Check sheet for the modelled part. Datum: model origin and axes. Units: mm. A direction names the side the tool comes from. Give positions to 0.01 mm unless a question says otherwise; leave off trailing zeros. Loops run counter-clockwise (first coordinate to the right, second up) from the corner with the lowest first, then second, coordinate; pieces in that order, holes last. Notation, with made-up numbers: M -28.5,18 L 23.5,18 A27 cw 23.5,54 Z; hole C -20,68.5 d3. An arc over 180 degrees is marked long. Write each question's results on one line, items separated by ' | '. Start each with the question number.
1. Go/stop test with flat-tipped pins: pin 1 (2.5 mm diameter, centred on x = -27, y = 6.5, fed in from -Z); pin 2 (0.6 mm diameter, centred on y = 6, z = -4, fed in from -X); pin 3 (6.5 mm diameter, centred on x = 27.5, y = 6, fed in from -Z). Record where each tip stops, or that it passes through.
2. Material ranges on line 1 along Y through (x, z) = (27.5, 5); line 2 along Z through (x, y) = (0, 8.75); line 3 along X through (y, z) = (4.75, -0.5), recorded low to high.
3. Sectioned sample at A-A on y = 7.5. Give the number of separate pieces and of enclosed holes in the cut face, and give its area (3 significant figures).
4. Tool access check on faces 5 (the cylindrical face through (-19.287, 0.752, -3.754)), 6 (the cylindrical face through (19.287, 0.752, -3.746)), 7 (the cylindrical face through (0, 14, -6)), 8 (the flat face through (0, 7, 1.5)), 9 (the flat face through (25.8, 5.8, 3.4)). Record the directions out of +Z, -Z, +X, -X, +Y, -Y that give a thin tool (end or side, any length) a straight path to the whole face; none if there is none.
5. Draft check along X on faces 1 (the flat face through (31, 5, -1)), 2 (the flat face through (35, 7, 3)), 3 (the cylindrical face through (-19, 8, -6)), 4 (the flat face through (-10, 7, 0)). Enter one of: pulls with the +X half, pulls with the -X half, needs draft (parallel to the pull), parting line crosses it, or undercut.
6. Sectioned sample at C-C on z = 5. Record the cut outline in (x, y), and give its area (3 significant figures).
7. Sectioned sample at D-D on y = 1.25. Record the cut outline in (x, z).
8. Sectioned sample at B-B on x = 27.5. Record the cut outline in (y, z).
```python
from build123d import *

# Parameters (mm, degrees)
SKETCH1_W                                           = 20
SKETCH1_H                                           = 3
BOSS_EXTRUDE1_DEPTH                                 = 15
CBORE_FOR_M4_HEX_SOCKET_HEAD_CAP_SCREW1_D           = 4.5
CBORE_FOR_M4_HEX_SOCKET_HEAD_CAP_SCREW1_CBORE_D     = 8
CBORE_FOR_M4_HEX_SOCKET_HEAD_CAP_SCREW1_CBORE_DEPTH = 4.4
FILLET1_R                                           = 2.5


with BuildPart() as part:
    # Sketch1 → Boss-Extrude1 (new body)
    with BuildSketch(Plane(origin=(0, 0, 0), x_dir=(1, 0, 0), z_dir=(0, 1, 0))):
        Polygon((-20, 6.5), (20, 6.5), (20, 1), (35, 1), (35, -8), (-35, -8), (-35, 1), (-20, 1), align=None)
        Rectangle(SKETCH1_W, SKETCH1_H, mode=Mode.SUBTRACT)
    extrude(amount=BOSS_EXTRUDE1_DEPTH)

    # CBORE for M4 Hex Socket Head Cap Screw1 (through all)
    with Locations(Plane(origin=(27.5, 7.5, -1), x_dir=(-1, 0, 0), z_dir=(0, 0, -1))):
        with Locations((0, 0), (55, 0)):
            CounterBoreHole(CBORE_FOR_M4_HEX_SOCKET_HEAD_CAP_SCREW1_D / 2, CBORE_FOR_M4_HEX_SOCKET_HEAD_CAP_SCREW1_CBORE_D / 2, CBORE_FOR_M4_HEX_SOCKET_HEAD_CAP_SCREW1_CBORE_DEPTH)

    # Fillet1
    fillet1_edges = [part.edges().sort_by_distance(p)[0] for p in [
        (-27.5, 0, -1),
        (-20, 0, -3.75),
        (-20, 7.5, -6.5),
        (20, 7.5, -6.5),
        (20, 7.5, -1),
        (-20, 7.5, -1),
        (27.5, 15, -1),
        (20, 15, -3.75),
        (0, 15, -6.5),
        (-20, 15, -3.75),
        (0, 0, -6.5),
        (-27.5, 15, -1),
        (20, 0, -3.75),
        (27.5, 0, -1),
    ]]
    fillet(fillet1_edges, radius=FILLET1_R)


solid = part.part
```
Output values:
1) pin 1: z = 3.4 | pin 2: x = -20 | pin 3: z = -1
2) line 1: 0 to 5.25, 9.75 to 15 | line 2: -6.5 to -1.5, 1.5 to 8 | line 3: -35 to -30.4, -24.6 to -10, 10 to 24.6, 30.4 to 35
3) separate pieces: 3 | enclosed holes: 1 | area: 678 mm2
4) face 5: -Z, -X, -Y | face 6: -Z, +X, -Y | face 7: -Z, +X, -X, +Y | face 8: +Y, -Y | face 9: -Z
5) face 1: needs draft | face 2: pulls with the +X half | face 3: pulls with the -X half | face 4: undercut
6) outline: M -35,0 L 35,0 L 35,15 L -35,15 Z; hole C -27.5,7.5 d4.5; hole C 27.5,7.5 d4.5 | area: 1,020 mm2
7) outline: M -35,-0.67 L -22.5,-0.67 A2.83 cw -19.67,-3.5 L -19.67,-4 A2.17 ccw -17.5,-6.17 L 17.5,-6.17 A2.17 ccw 19.67,-4 L 19.67,-3.5 A2.83 cw 22.5,-0.67 L 35,-0.67 L 35,8 L -35,8 Z; hole M -10,-1.5 L 10,-1.5 L 10,1.5 L -10,1.5 Z
8) outline: M 0,1.5 A2.5 ccw 2.5,-1 L 3.5,-1 L 3.5,3.4 L 5.25,3.4 L 5.25,8 L 0,8 Z; M 9.75,3.4 L 11.5,3.4 L 11.5,-1 L 12.5,-1 A2.5 ccw 15,1.5 L 15,8 L 9.75,8 Z
